Design review of the part built by this model. Coordinates are the model's own, in mm. Face numbers are marked on the shaded views. A direction names the side the tool comes from. Coordinates: 2 decimals unless noted, no trailing zeros. Loops run counter-clockwise (first coordinate to the right, second up) from the corner with the lowest first, then second, coordinate; pieces in that order, holes last. Notation, with made-up numbers: (73.25, -40) - (95.25, -40) arc R34 ccw to (95.25, -9) - close; hole circle Ø3 at (19.5, 86.25). An arc over 180 degrees is marked (long way). One line per question, with ' | ' between items.
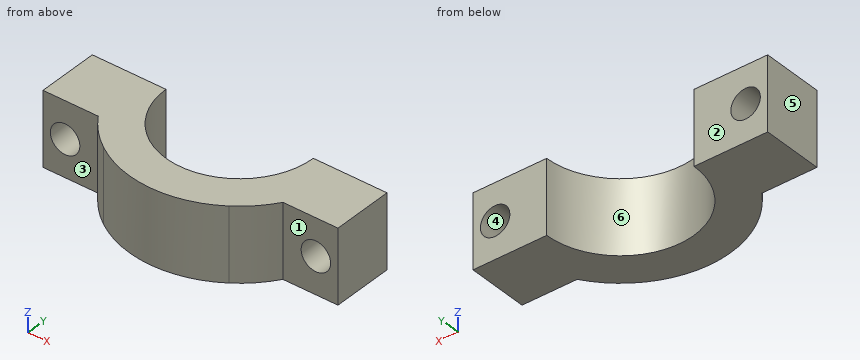
from build123d import *

# Parameters (mm, degrees)
BOSS_EXTRUDE1_DEPTH = 10


with BuildPart() as part:
    # Sketch1 → Boss-Extrude1 (new body)
    with BuildSketch(Plane.XY):
        with BuildLine():
            Line((-15, 0), (-10, 0))
            ThreePointArc((-10, 0), (0, -10), (10, 0))
            Line((10, 0), (15, 0))
            Line((15, 0), (20, 0))
            Line((20, 0), (20, -8.252048805))
            Line((20, -8.252048805), (12.52612033, -8.252048805))
            ThreePointArc((12.52612033, -8.252048805), (10.716124589, -10.495936061), (8.510293561, -12.352121417))
            ThreePointArc((8.510293561, -12.352121417), (0, -15), (-8.510293561, -12.352121417))
            ThreePointArc((-8.510293561, -12.352121417), (-10.697242908, -10.515179227), (-12.496376594, -8.297021877))
            Line((-12.496376594, -8.297021877), (-20, -8.297021877))
            Line((-20, -8.297021877), (-20, 0))
            Line((-20, 0), (-15, 0))
        make_face()
    extrude(amount=BOSS_EXTRUDE1_DEPTH)

    # Sketch7 → Ø4.0 (4) Diameter Hole2 (revolve, cut)
    with BuildSketch(Plane(origin=(17, 0, 5), x_dir=(0, 0, 1), z_dir=(1, 0, 0))):
        Polygon((0, 0), (0, 11.201721238), (2, 10), (2, 0), align=None)
    f_4_0_4_diameter_hole2 = revolve(axis=Axis((17, 6.35, 5), (0, -1, 0)), mode=Mode.SUBTRACT)

    # Mirror2: Ø4.0 (4) Diameter Hole2 across plane
    add(f_4_0_4_diameter_hole2.mirror(Plane(origin=(0, 0, 0), x_dir=(0, 0, 1), z_dir=(1, 0, 0))), mode=Mode.SUBTRACT)


solid = part.part
Q1. Tool access review of the marked faces 1 and 2: name each direction out of +Z, -Z, +X, -X, +Y, -Y from which nothing blocks a thin tool from reaching the whole face with its end or side.
Returned:
face 1: +Z, -Z, +X, -Y | face 2: +Z, -Z, +X, -X, +Y
Q2. For pin 1 (2.5 mm diameter, centred on x = -17, z = 5, fed in from -Y); pin 2 (5 mm diameter, centred on x = -15, y = -9, fed in from -Z), all flat-tipped, find the tip position at first contact; note any pin that passes through.
Returned:
pin 1: passes through | pin 2: stops at z = 0
Q3. Take a section at B-B (z = 5). Give the boundary of the cut face in (x, y), plus the area to 3 significant figures.
Returned:
outline: (-20, -8.3) - (-19, -8.3) - (-19, 0) - (-20, 0) - close; (-15, -8.3) - (-12.5, -8.3) arc R15 ccw to (12.53, -8.25) - (15, -8.25) - (15, 0) - (10, 0) arc R10 cw to (-10, 0) - (-15, 0) - close; (19, -8.25) - (20, -8.25) - (20, 0) - (19, 0) - close | area: 226 mm²
Q4. Draft analysis for pull direction X (two halves, no side actions). For the marked faces 3, 4, 5 and 6, state which applies: +X half, -X half, draft (parallel to the pull), parting line (faces both ways), or undercut.
Returned:
face 3: draft | face 4: undercut | face 5: -X half | face 6: undercut
Q5. Take a section at A-A (x = 17). Give the boundary of the cut face in (y, z).
Returned:
outline: (-8.25, 0) - (0, 0) - (0, 3) - (-8.25, 3) - close; (-8.25, 7) - (0, 7) - (0, 10) - (-8.25, 10) - close
Q6. To check wall thickness, follow line 1 along X through (y, z) = (-3.75, 5); line 2 along X through (y, z) = (-2.25, 6.25); line 3 along Y through (x, z) = (18, 3). State the ranges of each line that lie inside material, in increasing order.
Returned:
line 1: x = -20 to -19, -15 to -9.27, 9.27 to 15, 19 to 20 | line 2: x = -20 to -18.56, -15.44 to -9.74, 9.74 to 15.44, 18.56 to 20 | line 3: y = -8.25 to 0
Q7. Take a section at C-C (y = -1.5). Give the boundary of the cut face in (x, z), plus the area to 3 significant figures.
Returned:
outline: (-20, 0) - (-9.89, 0) - (-9.89, 10) - (-20, 10) - close; (9.89, 0) - (20, 0) - (20, 10) - (9.89, 10) - close; hole circle Ø4 at (-17, 5); hole circle Ø4 at (17, 5) | area: 177 mm²
Q8. Take a section at D-D (y = -9.5). Give the boundary of the cut face in (x, z).
Returned:
outline: (-11.61, 0) - (-3.12, 0) - (-3.12, 10) - (-11.61, 10) - close; (3.12, 0) - (11.61, 0) - (11.61, 10) - (3.12, 10) - close
